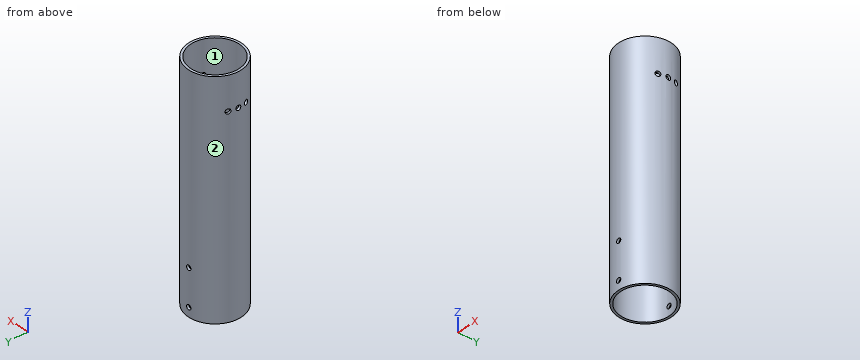
```python
from build123d import *

# Parameters (mm, degrees)
SKETCH_1_R          = 17.5
SKETCH_1_R_2        = 16
EXTRUDE_1_DEPTH     = 150
SKETCH_2_R          = 1.6
CUT_EXTRUDE_1_DEPTH = 25
SKETCH_5_R          = 1.6
CUT_EXTRUDE_3_DEPTH = 138.461236575
SKETCH_6_R          = 1.6
CUT_EXTRUDE_4_DEPTH = 25


with BuildPart() as part:
    # 草图1 → 凸台-拉伸1 (new body)
    with BuildSketch(Plane.XY):
        Circle(SKETCH_1_R)
        Circle(SKETCH_1_R_2, mode=Mode.SUBTRACT)
    extrude(amount=EXTRUDE_1_DEPTH)

    # 草图2 → 切除-拉伸1 (cut, symmetric)
    with BuildSketch(Plane(origin=(0, 0, 0), x_dir=(1, 0, 0), z_dir=(0, 1, 0))):
        with Locations(Location((0, -6, 0), (0, 0, 270))):
            Circle(SKETCH_2_R)
        with Locations(Location((0, -30, 0), (0, 0, 270))):
            Circle(SKETCH_2_R)
    extrude(amount=CUT_EXTRUDE_1_DEPTH, both=True, mode=Mode.SUBTRACT)

    # 草图5 → 切除-拉伸3 (cut, through all)
    with BuildSketch(Plane(origin=(24.979117188, 9.091655135, 128), x_dir=(0.3420201433256663, -0.9396926207859093, 0), z_dir=(0.9396926207859093, 0.3420201433256663, 0))):
        with Locations(Location((0, 0, 0), (0, 0, 180))):
            Circle(SKETCH_5_R)
    cut_extrude_3 = extrude(amount=-CUT_EXTRUDE_3_DEPTH, mode=Mode.SUBTRACT)

    # 镜向1: 切除-拉伸3 across plane
    add(cut_extrude_3.mirror(Plane(origin=(0, 0, 0), x_dir=(0, 0, 1), z_dir=(1, 0, 0))), mode=Mode.SUBTRACT)

    # 草图6 → 切除-拉伸4 (cut, symmetric)
    with BuildSketch(Plane(origin=(0, 0, 0), x_dir=(0, 0, -1), z_dir=(1, 0, 0))):
        with Locations((-128, 0)):
            Circle(SKETCH_6_R)
    extrude(amount=CUT_EXTRUDE_4_DEPTH, both=True, mode=Mode.SUBTRACT)


solid = part.part
```
Check sheet for the modelled part. Datum: model origin and axes. Units: mm. Face numbers are marked on the shaded views. Coordinates: 2 decimals unless noted, no trailing zeros. Write each loop counter-clockwise with the first axis right and the second up, starting at its lowest first coordinate (ties: lowest second). Pieces come first, ordered by that corner, then holes. Notation, with made-up numbers: (-28.5, 64) - (14.5, 64) arc R21 cw to (14.5, 94) - close; hole circle Ø1 at (16.25, 84.25). An arc over 180 degrees is marked (long way). One line per question, with ' | ' between items.
Item 1: Sectioned sample at B-B on x = 0. Record the boundary of the cut face in (y, z).
Determined:
outline: (-17.5, 0) - (-16, 0) - (-16, 4.4) - (-17.5, 4.4) - close; (-17.5, 7.6) - (-16, 7.6) - (-16, 28.4) - (-17.5, 28.4) - close; (-17.5, 31.6) - (-16, 31.6) - (-16, 150) - (-17.5, 150) - close; (16, 0) - (17.5, 0) - (17.5, 4.4) - (16, 4.4) - close; (16, 7.6) - (17.5, 7.6) - (17.5, 28.4) - (16, 28.4) - close; (16, 31.6) - (17.5, 31.6) - (17.5, 150) - (16, 150) - close
Item 2: Sectioned sample at A-A on y = 0. Record the boundary of the cut face in (x, z).
Determined:
outline: (-17.5, 0) - (-16, 0) - (-16, 126.4) - (-17.5, 126.4) - close; (-17.5, 129.6) - (-16, 129.6) - (-16, 150) - (-17.5, 150) - close; (16, 0) - (17.5, 0) - (17.5, 126.4) - (16, 126.4) - close; (16, 129.6) - (17.5, 129.6) - (17.5, 150) - (16, 150) - close
Item 3: Gauge pin test, flat ends, axial feed: P1, Ø1.5, axis at y = 4, z = 32, coming from the +X side; P2, Ø6, axis at y = 11, z = 84, coming from the -X side; P3, Ø5, axis at y = 0, z = 128, coming from the +X side; P4, Ø10, axis at y = -10.5, z = 121, coming from the -X side. Record the tip position at first contact, or that the pin passes through.
Determined:
P1: stops at x = 17.2 | P2: stops at x = -15.56 | P3: stops at x = 17.5 | P4: stops at x = -16.61
Item 4: Sectioned sample at D-D on z = 30. Record the boundary of the cut face in (x, y).
Determined:
outline: (-1.6, -17.43) - (-1.6, -15.92) arc R16 cw to (-1.6, 15.92) - (-1.6, 17.43) arc R17.5 ccw to start; (1.6, -17.43) arc R17.5 ccw to (1.6, 17.43) - (1.6, 15.92) arc R16 cw to (1.6, -15.92) - close
Item 5: Thickness scan on line 1 (Z direction, x = 0, y = 16.5); line 2 (X direction, y = 0, z = 130.5); line 3 (X direction, y = 16, z = 6). Record the ranges inside material, lowest first. Write a range as [from, to].
Determined:
line 1: z = [0, 4.4], [7.6, 28.4], [31.6, 150] | line 2: x = [-17.5, -16], [16, 17.5] | line 3: x = [-7.09, -1.6], [1.6, 7.09]
Item 6: Mould release check, pull along Y, two halves, no side actions. Record for the marked faces 1 and 2: pulls with the +Y half, pulls with the -Y half, needs draft (parallel to the pull), parting line crosses it, or undercut.
Determined:
face 1: undercut | face 2: parting line crosses it
Item 7: Sectioned sample at C-C on z = 128. Record the boundary of the cut face in (x, y), plus the area to 3 significant figures.
Determined:
outline: (-17.43, -1.6) arc R17.5 ccw to (-16.92, -4.46) - (-15.51, -3.94) arc R16 cw to (-15.92, -1.6) - close; (-17.43, 1.6) - (-15.92, 1.6) arc R16 cw to (-15.51, 3.94) - (-16.92, 4.46) arc R17.5 ccw to start; (-15.83, -7.46) arc R17.5 ccw to (15.83, -7.46) - (14.41, -6.95) arc R16 cw to (-14.41, -6.95) - close; (-15.83, 7.46) - (-14.41, 6.95) arc R16 cw to (14.41, 6.95) - (15.83, 7.46) arc R17.5 ccw to start; (15.51, -3.94) - (16.92, -4.46) arc R17.5 ccw to (17.43, -1.6) - (15.92, -1.6) arc R16 cw to start; (15.51, 3.94) arc R16 cw to (15.92, 1.6) - (17.43, 1.6) arc R17.5 ccw to (16.92, 4.46) - close | area: 129 mm2
